```python
from build123d import *

# Parameters (mm, degrees)
SKETCH1_W                    = 38.1
SKETCH1_H                    = 38.1
SKETCH1_W_2                  = 31.75
SKETCH1_H_2                  = 31.75
BOSS_EXTRUDE1_DEPTH          = 203.2
F_10_0_1935_DIAMETER_HOLE1_D = 4.9149
F_1_4_CLEARANCE_HOLE1_D      = 6.7564


with BuildPart() as part:
    # Sketch1 → Boss-Extrude1 (new body)
    with BuildSketch(Plane.XY):
        Rectangle(SKETCH1_W, SKETCH1_H)
        Rectangle(SKETCH1_W_2, SKETCH1_H_2, mode=Mode.SUBTRACT)
    extrude(amount=BOSS_EXTRUDE1_DEPTH)

    # #10 (0.1935) Diameter Hole1 (through all)
    with Locations(Plane.ZY.offset(19.05)):
        with Locations((22.225, 0), (66.675, 0), (136.525, 0), (180.975, 0)):
            Hole(F_10_0_1935_DIAMETER_HOLE1_D / 2)

    # 1/4 Clearance Hole1 (through all)
    with Locations(Plane(origin=(19.05, 0, 0), x_dir=(0, 0, -1), z_dir=(1, 0, 0))):
        with Locations((-101.6, 0)):
            Hole(F_1_4_CLEARANCE_HOLE1_D / 2)


solid = part.part
```
Work out the finished part from the listing and answer in its coordinate system (mm). A direction names the side the tool comes from. Round coordinates to 2 decimals unless told otherwise and drop trailing zeros. Write each loop counter-clockwise with the first axis right and the second up, starting at its lowest first coordinate (ties: lowest second). Pieces come first, ordered by that corner, then holes. Notation, with made-up numbers: (35, 43.5) -> (54, 43.5) arc R24 cw to (54, 55.5) -> close; hole circle Ø6 at (55, 63.25). An arc over 180 degrees is marked (long way). Write each question's results on one line, items separated by ' | '.
Q1. Section A-A, the plane z = 143.5 is taken. Write down the section's boundary in (x, y) (3 decimals).
Data:
outline: (-19.05, -19.05) -> (19.05, -19.05) -> (19.05, 19.05) -> (-19.05, 19.05) -> close; hole (-15.875, -15.875) -> (15.875, -15.875) -> (15.875, 15.875) -> (-15.875, 15.875) -> close
Q2. Section B-B, the plane x = 14 is taken. Write down the section's boundary in (y, z) (3 decimals).
Data:
outline: (-19.05, 0) -> (-15.875, 0) -> (-15.875, 203.2) -> (-19.05, 203.2) -> close; (15.875, 0) -> (19.05, 0) -> (19.05, 203.2) -> (15.875, 203.2) -> close
Q3. Flat-ended cylindrical pins translate along their axes: P1, Ø4.5, axis at y = 0, z = 22.225, coming from the -X side; P2, Ø11, axis at y = 0, z = 101.6, coming from the -X side. Find the tip coordinate at first contact, or state that the pin passes through.
Data:
P1: through | P2: x = -19.05
Q4. Section C-C, the plane z = 101.6 is taken. Write down the section's boundary in (x, y) (3 decimals).
Data:
outline: (-19.05, -19.05) -> (19.05, -19.05) -> (19.05, -3.378) -> (15.875, -3.378) -> (15.875, -15.875) -> (-15.875, -15.875) -> (-15.875, -3.378) -> (-19.05, -3.378) -> close; (-19.05, 3.378) -> (-15.875, 3.378) -> (-15.875, 15.875) -> (15.875, 15.875) -> (15.875, 3.378) -> (19.05, 3.378) -> (19.05, 19.05) -> (-19.05, 19.05) -> close
Q5. Determine the mould class of faces 3 (the flat face through (0, 19.05, 100)), 4 (the flat face through (19.05, 4, 100)), 5 (the cylindrical face through (-17.44, 0.11, 183.43)) for opening direction Y: released by +Y, released by -Y, zero draft, split by the parting line, or undercut.
Data:
face 3: released by +Y | face 4: zero draft | face 5: undercut
Q6. Which of the six approach directions +Z, -Z, +X, -X, +Y, -Y give full straight-line access (tool end or side, diameter ignored) to faces 1 (the flat face through (-19.05, 4, 100)), 2 (the flat face through (-15.875, 3.3, 100.2))?
Data:
face 1: +Z, -Z, -X, +Y, -Y | face 2: +Z, -Z
Q7. Straight lines are drawn through the part: line 1 along X through (y, z) = (3, 29) (3 decimals); line 2 along Y through (x, z) = (17.75, 101.6). For each, find the intervals that lie inside material, in ascending order. Write a range as [from, to].
Data:
line 1: [-19.05, -15.875], [15.875, 19.05] | line 2: [-19.05, -3.38], [3.38, 19.05]
